```python
from build123d import *

# Parameters (mm, degrees)
SKETCH1_W           = 65
SKETCH1_H           = 28
BOSS_EXTRUDE1_DEPTH = 10
CUT_EXTRUDE1_DEPTH  = 7
SKETCH3_W           = 10
SKETCH3_H           = 10
CUT_EXTRUDE2_DEPTH  = 7
BOSS_EXTRUDE5_DEPTH = 6
CUT_EXTRUDE6_DEPTH  = 1
SKETCH6_W           = 58
SKETCH6_H           = 3
SKETCH6_W_2         = 39
SKETCH6_H_2         = 3.5
CUT_EXTRUDE7_DEPTH  = 41
FILLET1_R           = 3


with BuildPart() as part:
    # Sketch1 → Boss-Extrude1 (new body)
    with BuildSketch(Plane(origin=(0, 0, 0), x_dir=(1, 0, 0), z_dir=(0, 1, 0))):
        Rectangle(SKETCH1_W, SKETCH1_H)
    extrude(amount=BOSS_EXTRUDE1_DEPTH)

    # Sketch2 → Cut-Extrude1 (cut)
    with BuildSketch(Plane(origin=(0, 10, 0), x_dir=(1, 0, 0), z_dir=(0, 1, 0))):
        Polygon((30, -11), (30, 11), (-30, 11), (-30, -11), (-30, -14), (30, -14), align=None)
    extrude(amount=-CUT_EXTRUDE1_DEPTH, mode=Mode.SUBTRACT)

    # Sketch3 → Cut-Extrude2 (cut)
    with BuildSketch(Plane(origin=(0, 3, 0), x_dir=(1, 0, 0), z_dir=(0, 1, 0))):
        with Locations((18, 0)):
            Rectangle(SKETCH3_W, SKETCH3_H)
    extrude(amount=-CUT_EXTRUDE2_DEPTH, mode=Mode.SUBTRACT)

    # Sketch4 → Boss-Extrude5 (add, symmetric)
    with BuildSketch(Plane(origin=(18, 0, 0), x_dir=(0, 0, -1), z_dir=(1, 0, 0))):
        with BuildLine():
            Line((-3.5, -3.5), (-2.121320344, -2.121320344))
            ThreePointArc((-2.121320344, -2.121320344), (0, 3), (2.121320344, -2.121320344))
            Line((2.121320344, -2.121320344), (3.5, -3.5))
            Line((3.5, -3.5), (3.5, 3.5))
            Line((3.5, 3.5), (-3.5, 3.5))
            Line((-3.5, 3.5), (-3.5, -3.5))
        make_face()
    extrude(amount=BOSS_EXTRUDE5_DEPTH, both=True)

    # Sketch5 → Cut-Extrude6 (cut)
    with BuildSketch(Plane.ZY.offset(-23)):
        with BuildLine():
            Line((-2.898275349, 0.1), (2.898275349, 0.1))
            ThreePointArc((2.898275349, 0.1), (0, 2.9), (-2.898275349, 0.1))
        make_face()
    cut_extrude6 = extrude(amount=-CUT_EXTRUDE6_DEPTH, mode=Mode.SUBTRACT)

    # Mirror1: Cut-Extrude6 across plane
    add(cut_extrude6.mirror(Plane(origin=(18, 0, 0), x_dir=(0, 0, 1), z_dir=(1, 0, 0))), mode=Mode.SUBTRACT)

    # Sketch6 → Cut-Extrude7 (cut)
    with BuildSketch(Plane(origin=(0, 3, 0), x_dir=(1, 0, 0), z_dir=(0, 1, 0))):
        with Locations((0, 7.5)):
            Rectangle(SKETCH6_W, SKETCH6_H)
        with Locations((-9.5, 2.25)):
            Rectangle(SKETCH6_W_2, SKETCH6_H_2)
        with Locations((-9.5, -5.25)):
            Rectangle(SKETCH6_W_2, SKETCH6_H_2)
        with Locations((0, -10.5)):
            Rectangle(SKETCH6_W, SKETCH6_H)
    extrude(amount=-CUT_EXTRUDE7_DEPTH, mode=Mode.SUBTRACT)

    # Fillet1
    fillet1_edges = [part.edges().sort_by_distance(p)[0] for p in [
        (32.5, 5, 14),
        (-32.5, 5, 14),
        (-32.5, 5, -14),
        (32.5, 5, -14),
    ]]
    fillet(fillet1_edges, radius=FILLET1_R)


solid = part.part
```
The model under review builds one solid part; all positions refer to its coordinate system, in mm. A direction names the side the tool comes from. Give positions to 0.01 mm unless a question says otherwise; leave off trailing zeros. Write each loop counter-clockwise with the first axis right and the second up, starting at its lowest first coordinate (ties: lowest second). Pieces come first, ordered by that corner, then holes. Notation, with made-up numbers: (-6.5, -33.75) -> (46.5, -33.75) arc R27 ccw to (46.5, -5.75) -> close; hole circle Ø8 at (56, -12). An arc over 180 degrees is marked (long way). Put each result on its own line as item: value.
(1) For pin 1 Ø0.5 at (x, z) = (23.5, 1.5) entering from +Y, flat-tipped, find the tip position at first contact; note if it passes through.
Results are:
pin 1: y = 3.5
(2) We need section D-D, the plane x = -28. Give the boundary of the cut face in (y, z).
Results are:
outline: (0, -14) -> (10, -14) -> (10, -11) -> (3, -11) -> (3, -9) -> (0, -9) -> close; (0, -6) -> (3, -6) -> (3, -4) -> (0, -4) -> close; (0, -0.5) -> (3, -0.5) -> (3, 3.5) -> (0, 3.5) -> close; (0, 7) -> (3, 7) -> (3, 9) -> (0, 9) -> close; (0, 12) -> (3, 12) -> (3, 14) -> (0, 14) -> close
(3) We need section B-B, the plane y = 8.25. Give the boundary of the cut face in (x, z).
Results are:
outline: (-32.5, -11) arc R3 ccw to (-29.5, -14) -> (29.5, -14) arc R3 ccw to (32.5, -11) -> (32.5, 11) arc R3 ccw to (30, 13.96) -> (30, -11) -> (-30, -11) -> (-30, 13.96) arc R3 ccw to (-32.5, 11) -> close
(4) The part is to be moulded in two halves that separate along Z. For faces 5 (the flat face through (24, -2, 3)), 6 (the flat face through (18, 2, 5)), 7 (the flat face through (0, 2, -9)), 8 (the cylindrical face through (-31.64, 5.07, -13.1)), say which applies: pulls with the +Z half, pulls with the -Z half, needs draft (parallel to the pull), parting line crosses it, or undercut.
Results are:
face 5: needs draft
face 6: undercut
face 7: undercut
face 8: pulls with the -Z half
(5) We need section A-A, the plane x = 18.5. Give the boundary of the cut face in (y, z), and give its area (3 significant figures).
Results are:
outline: (-3.5, -3.5) -> (3.5, -3.5) -> (3.5, 3.5) -> (-3.5, 3.5) -> (-2.12, 2.12) arc R3 cw (long way) to (-2.12, -2.12) -> close; (0, -14) -> (10, -14) -> (10, -11) -> (3, -11) -> (3, -9) -> (0, -9) -> close; (0, -6) -> (3, -6) -> (3, -5) -> (0, -5) -> close; (0, 5) -> (3, 5) -> (3, 9) -> (0, 9) -> close; (0, 12) -> (3, 12) -> (3, 14) -> (0, 14) -> close
area: 72.5 mm²
(6) We need section C-C, the plane z = -6.75. Give the boundary of the cut face in (x, y), and give its area (3 significant figures).
Results are:
outline: (-32.5, 0) -> (-29, 0) -> (-29, 3) -> (-30, 3) -> (-30, 10) -> (-32.5, 10) -> close; (29, 0) -> (32.5, 0) -> (32.5, 10) -> (30, 10) -> (30, 3) -> (29, 3) -> close
area: 56.0 mm²
(7) Tool access review of faces 1 (the flat face through (24, -2, -3)), 2 (the flat face through (18, -3, -3)), 3 (the flat face through (12, -2, -3)), 4 (the flat face through (23, 2, 4)): name each direction out of +Z, -Z, +X, -X, +Y, -Y from which nothing blocks a thin tool from reaching the whole face with its end or side.
Results are:
face 1: +Z, -Z, +X, -Y
face 2: +X, -X, -Y
face 3: +Z, -Z, -X, -Y
face 4: +Y, -Y
(8) To check wall thickness, follow probe 1 along X at (y, z) = (0.75, 9.5); probe 2 along X at (y, z) = (4.5, -3); probe 3 along Z at (x, y) = (3, 1.5). State the ranges of each line that lie inside material, in increasing order. Write a range as from..to.
Results are:
probe 1: -32.5..-29, 29..32.5
probe 2: -32.5..-30, 30..32.5
probe 3: -14..-9, -6..-4, -0.5..3.5, 7..9, 12..14
